```python
from build123d import *

# Parameters (mm, degrees)
F0_W     = 3.175
F0_H     = 160.30702
F1_DEPTH = 114.3
F2_W     = 146.1514011281
F2_H     = 3.175
F3_DEPTH = 12.7
F5_DEPTH = 25.4
F7_DEPTH = 25.4


with BuildPart() as f1:
    # F0 (on Top) → F1 (new body)
    with BuildSketch(Plane.XY):
        Rectangle(F0_W, F0_H)
    extrude(amount=F1_DEPTH)

    # F2 (on face) → F3 (join)
    with BuildSketch(Plane(origin=(-1.5875, 0, 0), x_dir=(0, -1, 0), z_dir=(-1, 0, 0))):
        with Locations((7.077809436, 112.7125)):
            Rectangle(F2_W, F2_H)
    extrude(amount=F3_DEPTH)

    # F4 (on face) → F5 (cut)
    with BuildSketch(Plane.XY.offset(114.3)):
        Polygon((-14.2875, 60.0979924202), (-1.5875, 65.9978911281), (-14.2875, 65.9978911281), align=None)
        Polygon((-14.2875, -80.15351), (-1.5875, -80.15351), (-14.2875, -65.9581273794), align=None)
    extrude(amount=-F5_DEPTH, mode=Mode.SUBTRACT)

    # F6 (on face) → F7 (cut)
    with BuildSketch(Plane.XY.offset(114.3)):
        with BuildLine():
            ThreePointArc((-4.7625, 50.3479417741), (-5.6924359697, 52.5930058044), (-7.9375, 53.5229417741))
            Line((-7.9375, 53.5229417741), (-7.9375, 47.1729417741))
            ThreePointArc((-7.9375, 47.1729417741), (-5.6924359697, 48.1028777439), (-4.7625, 50.3479417741))
        make_face()
        with BuildLine():
            ThreePointArc((-4.7625, -60.3558186897), (-5.6924359697, -58.1107546594), (-7.9375, -57.1808186897))
            Line((-7.9375, -57.1808186897), (-7.9375, -63.5308186897))
            ThreePointArc((-7.9375, -63.5308186897), (-5.6924359697, -62.60088272), (-4.7625, -60.3558186897))
        make_face()
        with BuildLine():
            Line((-7.9375, -63.5308186897), (-7.9375, -57.1808186897))
            ThreePointArc((-7.9375, -57.1808186897), (-11.1125, -60.3558186897), (-7.9375, -63.5308186897))
        make_face()
        with BuildLine():
            ThreePointArc((-4.7625, 0), (-5.6924359697, 2.2450640303), (-7.9375, 3.175))
            Line((-7.9375, 3.175), (-7.9375, -3.175))
            ThreePointArc((-7.9375, -3.175), (-5.6924359697, -2.2450640303), (-4.7625, 0))
        make_face()
        with BuildLine():
            Line((-7.9375, -3.175), (-7.9375, 3.175))
            ThreePointArc((-7.9375, 3.175), (-11.1125, 0), (-7.9375, -3.175))
        make_face()
        with BuildLine():
            Line((-7.9375, 47.1729417741), (-7.9375, 53.5229417741))
            ThreePointArc((-7.9375, 53.5229417741), (-11.1125, 50.3479417741), (-7.9375, 47.1729417741))
        make_face()
    extrude(amount=-F7_DEPTH, mode=Mode.SUBTRACT)


solid = f1.part
```
Could you check a few things on this model? Use its own coordinates, in mm. A direction names the side the tool comes from. Round coordinates to 2 decimals unless told otherwise and drop trailing zeros. Write each loop counter-clockwise with the first axis right and the second up, starting at its lowest first coordinate (ties: lowest second). Pieces come first, ordered by that corner, then holes.
(1) Suppose I cut it at A-A on y = -6. Write out the boundary of the cut face in (x, z) (1 decimal).
Findings below:
outline: (-14.3, 111.1) - (-1.6, 111.1) - (-1.6, 0) - (1.6, 0) - (1.6, 114.3) - (-14.3, 114.3) - close
(2) Which directions (+Z, -Z, +X, -X, +Y, -Y) give clear straight access to the entire face, cutting with the end or side of a thin tool? Please do faces 1 (the face through (-8, -6, 111.125)), 2 (the face through (-8.026, 63.007, 112.735)).
Findings below:
face 1: -Z, -X, +Y, -Y
face 2: +Z, -Z, -X, +Y
(3) For pin 1 (8 mm diameter, centred on y = -17.5, z = 22, fed in from -X); pin 2 (6.5 mm diameter, centred on x = -9, y = -35, fed in from -Z) (3 decimals); pin 3 (6 mm diameter, centred on x = -5.5, z = 32, fed in from -Y), each with a flat end and sliding along its axis, tell me the tip position at first contact or that it passes through.
Findings below:
pin 1: stops at x = -1.59
pin 2: stops at z = 111.125
pin 3: passes through
(4) If I drill on probe 1 along X at (y, z) = (-33, 8); probe 2 along Z at (x, y) = (-13, 22) (3 decimals), over which ranges is the centre line in solid material (lowest first)?
Findings below:
probe 1: x = -1.59 to 1.59
probe 2: z = 111.125 to 114.3
(5) Suppose I cut it at B-B on z = 103. Write out the boundary of the cut face in (x, y).
Findings below:
outline: (-1.59, -80.15) - (1.59, -80.15) - (1.59, 80.15) - (-1.59, 80.15) - close
